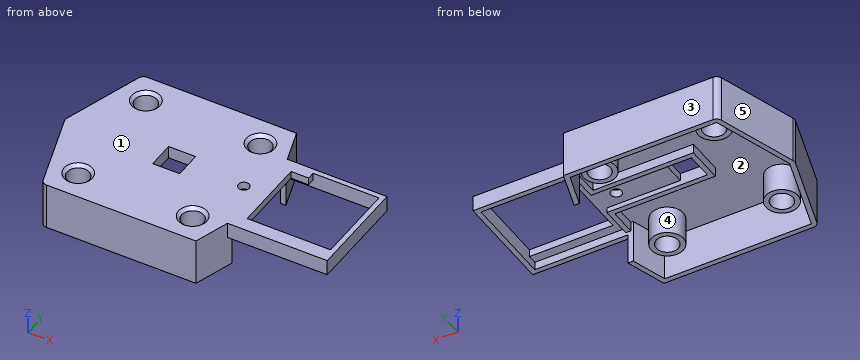
from build123d import *

# Parameters (mm, degrees)
BOSS_EXTRUDE1_DEPTH      = 10
BOSS_EXTRUDE1_DEPTH_BACK = 5
BOSS_EXTRUDE2_DEPTH      = 5
CUT_EXTRUDE1_DEPTH       = 68.390151358
BOSS_EXTRUDE3_DEPTH      = 4
SKETCH7_R                = 1.75
BOSS_EXTRUDE4_DEPTH      = 2.4
SKETCH8_R                = 3.5
BOSS_EXTRUDE5_DEPTH      = 1
SKETCH9_R                = 5.1
SKETCH9_R_2              = 3.5
BOSS_EXTRUDE6_DEPTH      = 9
CHAMFER1_SIZE            = 1
FILLET1_R                = 2


with BuildPart() as part:
    # Sketch2 → Boss-Extrude1 (new, two sides: drawn at the far end of the back side and taken through both)
    with BuildSketch(Plane.XY.offset(12).offset(-BOSS_EXTRUDE1_DEPTH_BACK)):
        Polygon((-24.532899998, 27.1), (-33.204899998, 0), (-24.532899998, -27.1), (24.532899998, -27.1), (33.204899998, 0), (24.532899998, 27.1), align=None)
        Polygon((-23.36497619, 25.5), (-31.52497619, 0), (-23.36497619, -25.5), (23.36497619, -25.5), (31.52497619, 0), (23.36497619, 25.5), align=None, mode=Mode.SUBTRACT)
    extrude(amount=BOSS_EXTRUDE1_DEPTH + BOSS_EXTRUDE1_DEPTH_BACK)

    # Sketch3 → Boss-Extrude2 (add)
    with BuildSketch(Plane.XY.offset(22)):
        Polygon((29.75, 16.1), (59.85, 16.1), (59.85, -16.1), (29.75, -16.1), (28.052899998, -16.1), (28.564899998, -14.5), (29.75, -14.5), (58.25, -14.5), (58.25, 14.5), (29.75, 14.5), (28.564899998, 14.5), (28.052899998, 16.1), align=None)
    extrude(amount=-BOSS_EXTRUDE2_DEPTH)

    # Sketch4 → Cut-Extrude1 (cut, through all)
    with BuildSketch(Plane(origin=(0, 0, 7), x_dir=(-1, 0, 0), z_dir=(0, 0, -1))):
        Polygon((-26.88497619, 14.5), (-28.564899998, 14.5), (-33.204899998, 0), (-28.564899998, -14.5), (-26.88497619, -14.5), (-31.52497619, 0), align=None)
    extrude(amount=-CUT_EXTRUDE1_DEPTH, mode=Mode.SUBTRACT)

    # Sketch5 → Boss-Extrude3 (add)
    with BuildSketch(Plane.XY.offset(22)):
        Polygon((29.25, 4.3), (29.25, 14), (29.25, 14.5), (27.65, 14.5), (27.65, 14), (27.65, 5.9), (-4.35, 5.9), (-4.35, -5.9), (27.65, -5.9), (27.65, -14), (27.65, -14.5), (29.25, -14.5), (29.25, -14), (29.25, -4.3), (-2.75, -4.3), (-2.75, 4.3), align=None)
    extrude(amount=-BOSS_EXTRUDE3_DEPTH)

    # Sketch7 → Boss-Extrude4 (add)
    with BuildSketch(Plane.XY.offset(22)):
        Polygon((37.25, 12.1), (37.25, 14.5), (29.25, 14.5), (29.25, 4.3), (5.85, 4.3), (5.85, -4.3), (29.25, -4.3), (29.25, -14.5), (58.25, -14.5), (58.25, -11.6), (31.65, -11.6), (31.65, 12.1), align=None)
        with Locations((23.75, 0)):
            Circle(SKETCH7_R, mode=Mode.SUBTRACT)
    extrude(amount=-BOSS_EXTRUDE4_DEPTH)

    # Sketch8 → Boss-Extrude5 (add)
    with BuildSketch(Plane.XY.offset(22)):
        Polygon((27.65, -5.9), (27.65, -14.5), (26.88497619, -14.5), (23.36497619, -25.5), (-23.36497619, -25.5), (-31.52497619, 0), (-23.36497619, 25.5), (23.36497619, 25.5), (26.88497619, 14.5), (27.65, 14.5), (27.65, 5.9), (-4.35, 5.9), (-4.35, -5.9), align=None)
        with Locations((-18.25, 18.25)):
            Circle(SKETCH8_R, mode=Mode.SUBTRACT)
        with Locations((18.25, 18.25)):
            Circle(SKETCH8_R, mode=Mode.SUBTRACT)
        with Locations((18.25, -18.25)):
            Circle(SKETCH8_R, mode=Mode.SUBTRACT)
        with Locations((-18.25, -18.25)):
            Circle(SKETCH8_R, mode=Mode.SUBTRACT)
    extrude(amount=-BOSS_EXTRUDE5_DEPTH)

    # Sketch9 → Boss-Extrude6 (add)
    # profile 1 of 4: a face of its own
    with BuildSketch(Plane(origin=(0, 0, 21), x_dir=(-1, 0, 0), z_dir=(0, 0, -1))):
        with Locations(Location((-18.25, 18.25, 0), (0, 0, 180))):
            Circle(SKETCH9_R)
        with Locations(Location((-18.25, 18.25, 0), (0, 0, 180))):
            Circle(SKETCH9_R_2, mode=Mode.SUBTRACT)
    # profile 2 of 4: a face of its own
    with BuildSketch(Plane(origin=(0, 0, 21), x_dir=(-1, 0, 0), z_dir=(0, 0, -1))):
        with Locations(Location((18.25, 18.25, 0), (0, 0, 180))):
            Circle(SKETCH9_R)
        with Locations(Location((18.25, 18.25, 0), (0, 0, 180))):
            Circle(SKETCH9_R_2, mode=Mode.SUBTRACT)
    # profile 3 of 4: a face of its own
    with BuildSketch(Plane(origin=(0, 0, 21), x_dir=(-1, 0, 0), z_dir=(0, 0, -1))):
        with Locations(Location((18.25, -18.25, 0), (0, 0, 180))):
            Circle(SKETCH9_R)
        with Locations(Location((18.25, -18.25, 0), (0, 0, 180))):
            Circle(SKETCH9_R_2, mode=Mode.SUBTRACT)
    # profile 4 of 4: a face of its own
    with BuildSketch(Plane(origin=(0, 0, 21), x_dir=(-1, 0, 0), z_dir=(0, 0, -1))):
        with Locations(Location((-18.25, -18.25, 0), (0, 0, 180))):
            Circle(SKETCH9_R)
        with Locations(Location((-18.25, -18.25, 0), (0, 0, 180))):
            Circle(SKETCH9_R_2, mode=Mode.SUBTRACT)
    extrude(amount=BOSS_EXTRUDE6_DEPTH)

    # Chamfer1
    chamfer1_edges = [part.edges().sort_by_distance(p)[0] for p in [
        (-21.75, -18.25, 22),
        (14.75, -18.25, 22),
        (14.75, 18.25, 22),
        (-21.75, 18.25, 22),
    ]]
    chamfer(chamfer1_edges, length=CHAMFER1_SIZE - 0.0001)  # a hair under: the kernel refuses the full size

    # Fillet1
    fillet1_edges = [part.edges().sort_by_distance(p)[0] for p in [
        (-24.532899998, -27.1, 14.5),
        (-33.204899998, 0, 14.5),
        (-24.532899998, 27.1, 14.5),
    ]]
    fillet(fillet1_edges, radius=FILLET1_R)


solid = part.part
Could you check a few things on this model? Use its own coordinates, in mm. Face numbers are marked on the shaded views. A direction names the side the tool comes from. Give positions to 0.01 mm unless a question says otherwise; leave off trailing zeros. Write each loop counter-clockwise with the first axis right and the second up, starting at its lowest first coordinate (ties: lowest second). Pieces come first, ordered by that corner, then holes. Notation, with made-up numbers: (-7.75, -18) -> (39.25, -18) arc R30 cw to (39.25, 20) -> close; hole circle Ø6 at (-9.5, 32). An arc over 180 degrees is marked (long way). Answer as CSV lines item,"result". Start each with the question number.
(1) If we section it at D-D, the plane y = -18.25: Write out the boundary of the cut face in (x, z).
(2) If we section it at A-A, the plane z = 14: Give the number of separate pieces and of enclosed holes in the cut face, and give its area (3 significant figures).
(3) If we mould it in two halves opening along Y, with no side actions, what happens to the marked faces 1, 2 and 3? For each: +Y half, -Y half, draft (parallel to the pull), parting line (faces both ways), or undercut.
(4) Which directions (+Z, -Z, +X, -X, +Y, -Y) give clear straight access to the entire face, cutting with the end or side of a thin tool? Please do the marked faces 4 and 5.
(5) If we section it at C-C, the plane x = 45.5: Write out the boundary of the cut face in (y, z).
(6) Please list where these lines run through material, in increasing order: line 1 (Y direction, x = 18.25, z = 15); line 2 (Y direction, x = 2, z = 17.5); line 3 (X direction, y = -18.25, z = 17).
(7) If we section it at B-B, the plane x = -18.25: Write out the boundary of the cut face in (y, z), and give its area (3 significant figures).
(8) I'm going to push flat-ended pins straight in: pin 1 Ø5 at (x, y) = (-16.5, 16.5) entering from -Z; pin 2 Ø5.5 at (x, z) = (38, 20) entering from +Y; pin 3 Ø4 at (y, z) = (-18.5, 16) entering from +X; pin 4 Ø6.5 at (x, y) = (-18.25, 18.25) entering from +Z. Where does each tip first touch, or does it pass through?
Answer list:
1,outline,"(-27.36, 7) -> (-25.68, 7) -> (-25.68, 21) -> (-23.35, 21) -> (-23.35, 12) -> (-21.75, 12) -> (-21.75, 21) -> (-22.75, 22) -> (-27.36, 22) -> close; (-14.75, 12) -> (-13.15, 12) -> (-13.15, 21) -> (13.15, 21) -> (13.15, 12) -> (14.75, 12) -> (14.75, 21) -> (13.75, 22) -> (-13.75, 22) -> (-14.75, 21) -> close; (21.75, 12) -> (23.35, 12) -> (23.35, 21) -> (25.68, 21) -> (25.68, 7) -> (27.36, 7) -> (27.36, 22) -> (22.75, 22) -> (21.75, 21) -> close"
2,separate pieces,"5"
2,enclosed holes,"4"
2,area,"453 mm^2"
3,face 1,"draft"
3,face 2,"undercut"
3,face 3,"+Y half"
4,face 4,"-Z"
4,face 5,"+Z, -Z, -X, +Y"
5,outline,"(-16.1, 17) -> (-14.5, 17) -> (-14.5, 19.6) -> (-11.6, 19.6) -> (-11.6, 22) -> (-16.1, 22) -> close; (14.5, 17) -> (16.1, 17) -> (16.1, 22) -> (14.5, 22) -> close"
6,line 1,"-27.1 to -25.5, -23.35 to -21.75, -14.75 to -13.15, 13.15 to 14.75, 21.75 to 23.35, 25.5 to 27.1"
6,line 2,"-27.1 to -25.5, 25.5 to 27.1"
6,line 3,"-27.36 to -25.68, -23.35 to -21.75, -14.75 to -13.15, 13.15 to 14.75, 21.75 to 23.35, 25.68 to 27.36"
7,outline,"(-27.1, 7) -> (-25.5, 7) -> (-25.5, 21) -> (-23.35, 21) -> (-23.35, 12) -> (-21.75, 12) -> (-21.75, 21) -> (-22.75, 22) -> (-27.1, 22) -> close; (-14.75, 12) -> (-13.15, 12) -> (-13.15, 21) -> (13.15, 21) -> (13.15, 12) -> (14.75, 12) -> (14.75, 21) -> (13.75, 22) -> (-13.75, 22) -> (-14.75, 21) -> close; (21.75, 12) -> (23.35, 12) -> (23.35, 21) -> (25.5, 21) -> (25.5, 7) -> (27.1, 7) -> (27.1, 22) -> (22.75, 22) -> (21.75, 21) -> close"
7,area,"141 mm^2"
8,pin 1,"z = 12"
8,pin 2,"y = 16.1"
8,pin 3,"x = 27.92"
8,pin 4,"through"
